from build123d import *

# Parameters (mm, degrees)
SKETCH1_W           = 58.42
SKETCH1_H           = 58.42
BOSS_EXTRUDE1_DEPTH = 3.81
SKETCH2_R           = 1.5999968
SKETCH2_R_2         = 1.6
CUT_EXTRUDE1_DEPTH  = 3.81
SKETCH5_W           = 10.202183674
SKETCH5_H           = 29.21
CUT_EXTRUDE3_DEPTH  = 3.81


with BuildPart() as part:
    # Sketch1 → Boss-Extrude1 (new body)
    with BuildSketch(Plane.XY):
        Rectangle(SKETCH1_W, SKETCH1_H)
    extrude(amount=BOSS_EXTRUDE1_DEPTH)

    # Sketch2 → Cut-Extrude1 (cut)
    with BuildSketch(Plane.XY.offset(3.81)):
        with Locations((-25.400000617, 25.400000617)):
            Circle(SKETCH2_R)
        with Locations((25.400000617, 25.400000617)):
            Circle(SKETCH2_R_2)
        with Locations((-25.400000617, -25.400000617)):
            Circle(SKETCH2_R_2)
        with Locations((25.400000617, -25.400000617)):
            Circle(SKETCH2_R_2)
    extrude(amount=-CUT_EXTRUDE1_DEPTH, mode=Mode.SUBTRACT)

    # Sketch5 → Cut-Extrude3 (cut)
    with BuildSketch(Plane.XY.offset(3.81)):
        with Locations((0.091911565, 14.605)):
            Rectangle(SKETCH5_W, SKETCH5_H)
    extrude(amount=-CUT_EXTRUDE3_DEPTH, mode=Mode.SUBTRACT)


solid = part.part
Work out the finished part from the listing and answer in its coordinate system (mm). A direction names the side the tool comes from. Give positions to 0.01 mm unless a question says otherwise; leave off trailing zeros. Loops run counter-clockwise (first coordinate to the right, second up) from the corner with the lowest first, then second, coordinate; pieces in that order, holes last. Notation, with made-up numbers: (-20.75, 6.5) -> (-15.75, 6.5) arc R26 ccw to (-15.75, 20.5) -> close; hole circle Ø8 at (-26.75, 26.25). An arc over 180 degrees is marked (long way). Use a Markdown table: item, result. Add a question column.
1. Find the intervals of material crossed by probe 1 along X at (y, z) = (-25.4, 2.9); probe 2 along X at (y, z) = (-26, 2.1), in increasing order.
2. Determine the mould class of faces 1 (the flat face through (0, 0, 2)), 2 (the flat face through (0, -29.21, 2)), 3 (the cylindrical face through (-24.66, 23.98, 1.93)), 4 (the flat face through (0, -6, 3.81)) for opening direction Y: released by +Y, released by -Y, zero draft, split by the parting line, or undercut.
3. Section B-B on x = 25.4 is taken. Determine the outline of the cut face in (y, z), and give its area (3 significant figures).
4. For faces 5 (the flat face through (-5.009, 14, 2)), 6 (the flat face through (-29.21, 0, 2)), determine the directions among +Z, -Z, +X, -X, +Y, -Y from which every point of the face is accessible in a straight line to the end or side of a thin tool.
5. Section A-A on y = 11.5 is taken. Determine the outline of the cut face in (x, z).
6. Section D-D on z = 0.6 is taken. Determine the outline of the cut face in (x, y).
Results below:
| question | item | result |
|---|---|---|
| 1 | probe 1 | x = -29.21 to -27, -23.8 to 23.8, 27 to 29.21 |
| 1 | probe 2 | x = -29.21 to -26.88, -23.92 to 23.92, 26.88 to 29.21 |
| 2 | face 1 | released by +Y |
| 2 | face 2 | released by -Y |
| 2 | face 3 | undercut |
| 2 | face 4 | zero draft |
| 3 | outline | (-29.21, 0) -> (-27, 0) -> (-27, 3.81) -> (-29.21, 3.81) -> close; (-23.8, 0) -> (23.8, 0) -> (23.8, 3.81) -> (-23.8, 3.81) -> close; (27, 0) -> (29.21, 0) -> (29.21, 3.81) -> (27, 3.81) -> close |
| 3 | area | 198 mm^2 |
| 4 | face 5 | +Z, -Z, +Y |
| 4 | face 6 | +Z, -Z, -X, +Y, -Y |
| 5 | outline | (-29.21, 0) -> (-5.01, 0) -> (-5.01, 3.81) -> (-29.21, 3.81) -> close; (5.19, 0) -> (29.21, 0) -> (29.21, 3.81) -> (5.19, 3.81) -> close |
| 6 | outline | (-29.21, -29.21) -> (29.21, -29.21) -> (29.21, 29.21) -> (5.19, 29.21) -> (5.19, 0) -> (-5.01, 0) -> (-5.01, 29.21) -> (-29.21, 29.21) -> close; hole circle Ø3.2 at (-25.4, -25.4); hole circle Ø3.2 at (-25.4, 25.4); hole circle Ø3.2 at (25.4, -25.4); hole circle Ø3.2 at (25.4, 25.4) |
